```python
from build123d import *

# Parameters (mm, degrees)
SKETCH1_R                 = 18.4
BOSS_EXTRUDE1_DEPTH       = 22
M3X0_5_TAPPED_HOLE1_D     = 2.5
M3X0_5_TAPPED_HOLE1_DEPTH = 7.62
M3X0_5_TAPPED_HOLE1_TIP   = 0.751075774
SKETCH6_R                 = 17.25
BOSS_EXTRUDE2_DEPTH       = 30
SKETCH7_R                 = 3
BOSS_EXTRUDE3_DEPTH       = 22
CUT_EXTRUDE1_DEPTH        = 12
SKETCH9_R                 = 6
BOSS_EXTRUDE4_DEPTH       = 6.5


with BuildPart() as part:
    # Sketch1 → Boss-Extrude1 (new body)
    with BuildSketch(Plane.XY):
        Circle(SKETCH1_R)
    extrude(amount=BOSS_EXTRUDE1_DEPTH)

    # M3x0.5 Tapped Hole1
    with Locations(Plane.XY.offset(22)):
        with Locations((-13.423393759, 7.75), (0, 15.5), (13.423393759, 7.75), (13.423393759, -7.75), (0, -15.5), (-13.423393759, -7.75)):
            Hole(M3X0_5_TAPPED_HOLE1_D / 2, depth=M3X0_5_TAPPED_HOLE1_DEPTH)
            with Locations((0, 0, -(M3X0_5_TAPPED_HOLE1_DEPTH + M3X0_5_TAPPED_HOLE1_TIP / 2))):  # 118° drill point
                Cone(0, M3X0_5_TAPPED_HOLE1_D / 2, M3X0_5_TAPPED_HOLE1_TIP, mode=Mode.SUBTRACT)

    # Sketch6 → Boss-Extrude2 (add)
    with BuildSketch(Plane(origin=(0, 0, 0), x_dir=(-1, 0, 0), z_dir=(0, 0, -1))):
        Circle(SKETCH6_R)
    extrude(amount=BOSS_EXTRUDE2_DEPTH)

    # Sketch7 → Boss-Extrude3 (add)
    with BuildSketch(Plane.XY.offset(22)):
        with Locations((7, 0)):
            Circle(SKETCH7_R)
    extrude(amount=BOSS_EXTRUDE3_DEPTH)

    # Sketch8 → Cut-Extrude1 (cut)
    with BuildSketch(Plane.XY.offset(44)):
        with BuildLine():
            Line((5.2, 2.4), (8.8, 2.4))
            ThreePointArc((8.8, 2.4), (7, 3), (5.2, 2.4))
        make_face()
    extrude(amount=-CUT_EXTRUDE1_DEPTH, mode=Mode.SUBTRACT)

    # Sketch9 → Boss-Extrude4 (add)
    with BuildSketch(Plane.XY.offset(22)):
        with Locations((7, 0)):
            Circle(SKETCH9_R)
    extrude(amount=BOSS_EXTRUDE4_DEPTH)


solid = part.part
```
The model under review builds one solid part; all positions refer to its coordinate system, in mm. A direction names the side the tool comes from. Round coordinates to 2 decimals unless told otherwise and drop trailing zeros. Order: outer loops, then holes, each group sorted by start corner. A loop starts at its lowest first (then second) coordinate and runs counter-clockwise, first axis right, second up. Notation, with made-up numbers: (-22, -21) -> (10, -21) arc R17 ccw to (10, 11) -> close; hole circle Ø9 at (2.5, 47.25). An arc over 180 degrees is marked (long way). One line per item, written item: value. Start each with the question number.
Q1. Mouldability with a two-part tool opening along X and no side actions: class faces 5 (the face through (1, 0, 25)), 6 (the face through (-0.672, 16.554, 18.137)), 7 (the face through (0, 0, -30)) as released by +X, released by -X, zero draft, split by the parting line, or undercut.
Q2. Take a section at A-A (y = 0). Write out the cut boundary in (x, z), and give its area (3 significant figures).
Q3. Clearance check with flat-ended pins moving along their axes: pin 1 Ø1.8 at (x, z) = (7, 39) entering from +Y; pin 2 Ø10 at (y, z) = (10.5, -18.5) entering from -X; pin 3 Ø5 at (x, z) = (-6, -6) entering from +Y. State where each tip first meets the part, or that it passes through.
Q4. Take a section at C-C (x = 7). Write out the cut boundary in (y, z), and give its area (3 significant figures).
Q5. Wall thickness on line 1 (Y direction, x = 0, z = 18.5); line 2 (Y direction, x = 1, z = 16); line 3 (X direction, y = 7, z = 17): over which ranges is each line inside the solid? List them lowest first.
Q6. Take a section at B-B (z = -24). Write out the cut boundary in (x, y).
Q7. Machinability: for faces 1 (the face through (-12.43, 6.99, 18.14)), 2 (the face through (7, 0, 44)), 3 (the face through (-16.453, 5.181, -14.79)), 4 (the face through (7, 2.4, 38)), which of the approach directions +Z, -Z, +X, -X, +Y, -Y give a long, thin tool a straight path to every point of the face, cutting with its end or side? Answer none if there is none.
Q8. Take a section at D-D (y = 10). Write out the cut boundary in (x, z).
Reported:
1. face 5: split by the parting line
1. face 6: undercut
1. face 7: zero draft
2. outline: (-18.4, 0) -> (-17.25, 0) -> (-17.25, -30) -> (17.25, -30) -> (17.25, 0) -> (18.4, 0) -> (18.4, 22) -> (13, 22) -> (13, 28.5) -> (10, 28.5) -> (10, 44) -> (4, 44) -> (4, 28.5) -> (1, 28.5) -> (1, 22) -> (-18.4, 22) -> close
2. area: 2,020 mm2
3. pin 1: stops at y = 2.4
3. pin 2: stops at x = -16.35
3. pin 3: stops at y = 16.89
4. outline: (-17.02, 0) -> (-15.77, 0) -> (-15.77, -30) -> (15.77, -30) -> (15.77, 0) -> (17.02, 0) -> (17.02, 22) -> (6, 22) -> (6, 28.5) -> (3, 28.5) -> (3, 32) -> (2.4, 32) -> (2.4, 44) -> (-3, 44) -> (-3, 28.5) -> (-6, 28.5) -> (-6, 22) -> (-17.02, 22) -> close
4. area: 1,860 mm2
5. line 1: y = -18.4 to -16.75, -14.25 to 14.25, 16.75 to 18.4
5. line 2: y = -18.37 to -16.25, -14.75 to 14.75, 16.25 to 18.37
5. line 3: x = -17.02 to -14.42, -12.42 to 12.42, 14.42 to 17.02
6. outline: circle Ø34.5 at (0, 0)
7. face 1: +Z
7. face 2: +Z, +X, -X, +Y, -Y
7. face 3: -Z
7. face 4: +Z, +X, -X, +Y
8. outline: (-15.45, 0) -> (-14.06, 0) -> (-14.06, -30) -> (14.06, -30) -> (14.06, 0) -> (15.45, 0) -> (15.45, 22) -> (-15.45, 22) -> close
